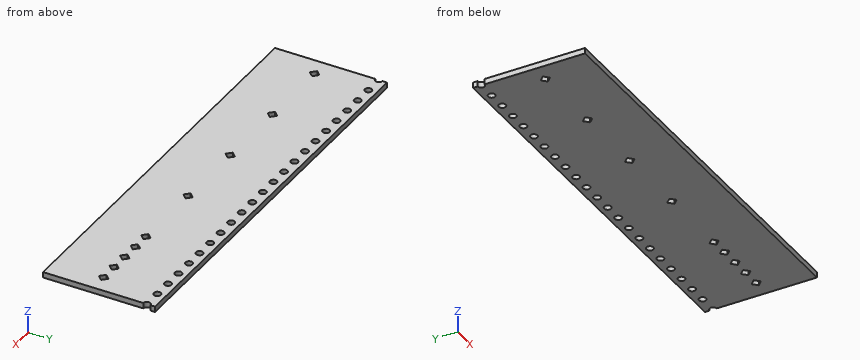
from build123d import *

# Parameters (mm, degrees)
TOP_SKETCH_W                   = 88
TOP_SKETCH_H                   = 24
THICKNESS_EXTRUDE_DEPTH        = 1.2
PIN_HOLE_SKETCH_R              = 0.75
FIRST_PIN_HOLE_CUT_DEPTH       = 92.221927189
PIN_HOLE_PATTERN_COUNT         = 23
PIN_HOLE_PATTERN_PITCH         = 4
MARKER_CUT_DEPTH               = 92.221927189
COMPONENT_MARKER_PATTERN_COUNT = 4
COMPONENT_MARKER_PATTERN_PITCH = 4
PIN_HOLE_MARKER_PATTERN_COUNT  = 6
PIN_HOLE_MARKER_PATTERN_PITCH  = 16


with BuildPart() as part:
    # Top Sketch → Thickness Extrude (new body)
    with BuildSketch(Plane.XY):
        with Locations((-44, -12)):
            Rectangle(TOP_SKETCH_W, TOP_SKETCH_H)
    extrude(amount=-THICKNESS_EXTRUDE_DEPTH)

    # Pin Hole Sketch → First Pin Hole Cut (cut, through all)
    with BuildSketch(Plane.XY):
        with Locations((0, -1.75)):
            Circle(PIN_HOLE_SKETCH_R)
    first_pin_hole_cut = extrude(amount=-FIRST_PIN_HOLE_CUT_DEPTH, mode=Mode.SUBTRACT)

    # Pin Hole Pattern: First Pin Hole Cut ×23
    with Locations(*[(-i * PIN_HOLE_PATTERN_PITCH, 0, 0) for i in range(1, PIN_HOLE_PATTERN_COUNT)]):
        add(first_pin_hole_cut, mode=Mode.SUBTRACT)

    # Marker Sketch → Marker Cut (cut, through all)
    with BuildSketch(Plane.XY):
        Polygon((-4, -12.25), (-5, -13.25), (-4, -14.25), (-3, -13.25), align=None)
    marker_cut = extrude(amount=-MARKER_CUT_DEPTH, mode=Mode.SUBTRACT)

    # Component Marker Pattern: Marker Cut ×4
    with Locations(*[(-i * COMPONENT_MARKER_PATTERN_PITCH, 0, 0) for i in range(1, COMPONENT_MARKER_PATTERN_COUNT)]):
        add(marker_cut, mode=Mode.SUBTRACT)

    # Pin Hole Marker Pattern: Marker Cut ×6
    with Locations(*[(-i * PIN_HOLE_MARKER_PATTERN_PITCH, 0, 0) for i in range(1, PIN_HOLE_MARKER_PATTERN_COUNT)]):
        add(marker_cut, mode=Mode.SUBTRACT)


solid = part.part
Can you work these out from the model? Positions are in its coordinate system, mm. Give positions to 0.01 mm unless a question says otherwise; leave off trailing zeros. Order: outer loops, then holes, each group sorted by start corner. A loop starts at its lowest first (then second) coordinate and runs counter-clockwise, first axis right, second up. Notation, with made-up numbers: (-37.75, 20.5) - (16.25, 20.5) arc R23 ccw to (16.25, 38.5) - close; hole circle Ø4 at (-10, -32.75). An arc over 180 degrees is marked (long way). Write each question's results on one line, items separated by ' | '.
1) I'm going to push flat-ended pins straight in: pin 1 Ø0.9 at (x, y) = (-12, -1.75) entering from -Z; pin 2 Ø2.5 at (x, y) = (-72, -1.75) entering from -Z. Where does each tip first touch, or does it pass through?
Final values:
pin 1: passes through | pin 2: stops at z = -1.2
2) Please list where these lines run through material, in increasing order: line 1 along Y through (x, z) = (-60, -0.8); line 2 along Y through (x, z) = (-52.5, -0.3); line 3 along Y through (x, z) = (-43.5, -0.25). Write a range as [from, to].
Final values:
line 1: y = [-24, -2.5], [-1, 0] | line 2: y = [-24, -13.75], [-12.75, -2.31], [-1.19, 0] | line 3: y = [-24, -2.31], [-1.19, 0]
3) Suppose I cut it at A-A, the plane x = -24. Write out the boundary of the cut face in (y, z), then the cut area to 3 significant figures.
Final values:
outline: (-24, -1.2) - (-2.5, -1.2) - (-2.5, 0) - (-24, 0) - close; (-1, -1.2) - (0, -1.2) - (0, 0) - (-1, 0) - close | area: 27.0 mm^2
